Study the drawing (mm; zero at the part's minimum x, y, z) and answer. A direction names the side the tool comes from. Round coordinates to 2 decimals unless told otherwise and drop trailing zeros. Write each loop counter-clockwise with the first axis right and the second up, starting at its lowest first coordinate (ties: lowest second). Pieces come first, ordered by that corner, then holes. Notation, with made-up numbers: (49.5, 78.5) -> (107.5, 78.5) arc R19 ccw to (107.5, 97.5) -> close; hole circle Ø10 at (-39.75, 57). An arc over 180 degrees is marked (long way). Return JSON: item names as keys, results as strings.
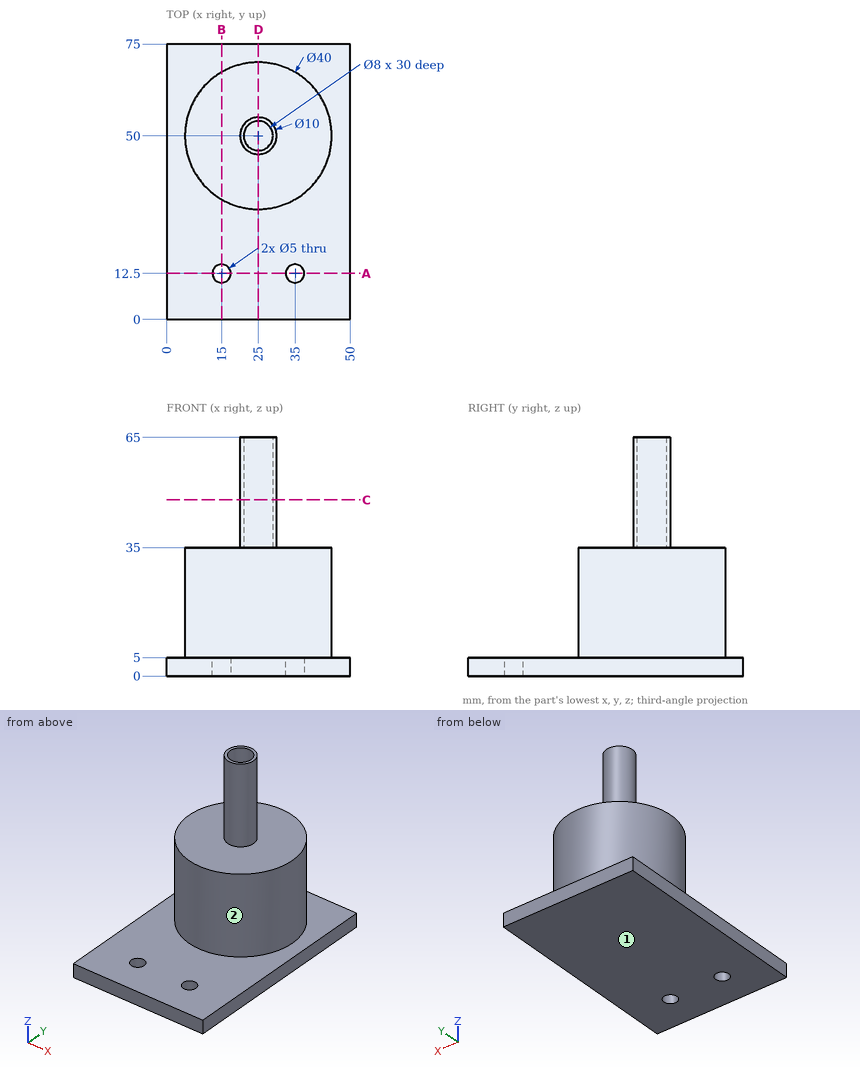
Item 1: Flat-ended cylindrical pins translate along their axes: pin 1 (8 mm diameter, centred on x = 35, z = 11.5, fed in from -Y); pin 2 (6 mm diameter, centred on y = 34, z = 18.5, fed in from -X); pin 3 (12 mm diameter, centred on y = 54.5, z = 24.5, fed in from -X). Find the tip coordinate at first contact, or state that the pin passes through.
Worked answers:
{"pin 1": "stops at y = 30.92", "pin 2": "stops at x = 9.8", "pin 3": "stops at x = 5"}
Item 2: Section C-C (z = 48) is taken. Give the vertices of the cut face in (x, y), then the cut area to 3 significant figures.
Worked answers:
{"outline": "circle Ø10 at (25, 50); hole circle Ø8 at (25, 50)", "area": "28.3 mm2"}
Item 3: A tool of negligible diameter and unlimited length cuts with its end or side. For the marked faces 1 and 2, from which of +Z, -Z, +X, -X, +Y, -Y can it reach the whole face along a straight path? Write none if from no direction.
Worked answers:
{"face 1": "-Z, +X, -X, +Y, -Y", "face 2": "+Z"}
Item 4: Section A-A (y = 12.5) is taken. Give the vertices of the cut face in (x, z).
Worked answers:
{"outline": "(0, 0) -> (12.5, 0) -> (12.5, 5) -> (0, 5) -> close; (17.5, 0) -> (32.5, 0) -> (32.5, 5) -> (17.5, 5) -> close; (37.5, 0) -> (50, 0) -> (50, 5) -> (37.5, 5) -> close"}
Item 5: Section D-D (x = 25) is taken. Give the vertices of the cut face in (y, z), then the cut area to 4 significant figures.
Worked answers:
{"outline": "(0, 0) -> (75, 0) -> (75, 5) -> (70, 5) -> (70, 35) -> (55, 35) -> (55, 65) -> (54, 65) -> (54, 35) -> (46, 35) -> (46, 65) -> (45, 65) -> (45, 35) -> (30, 35) -> (30, 5) -> (0, 5) -> close", "area": "1,635 mm2"}
Item 6: Section B-B (x = 15) is taken. Give the vertices of the cut face in (y, z).
Worked answers:
{"outline": "(0, 0) -> (10, 0) -> (10, 5) -> (0, 5) -> close; (15, 0) -> (75, 0) -> (75, 5) -> (67.32, 5) -> (67.32, 35) -> (32.68, 35) -> (32.68, 5) -> (15, 5) -> close"}
Item 7: Straight lines are drawn through the part: L1, parallel to Y at x = 25, z = 57; L2, parallel to Y at x = 15, z = 3; L3, parallel to Z at x = 11.5, y = 42. For each, find the intervals that lie inside material, in ascending order. Write a range as [from, to].
Worked answers:
{"L1": "y = [45, 46], [54, 55]", "L2": "y = [0, 10], [15, 75]", "L3": "z = [0, 35]"}
